Source: CAD feature listing. Evaluate the final solid. Frame: model axes, mm. A direction names the side the tool comes from. Round coordinates to 2 decimals unless told otherwise and drop trailing zeros. Order: outer loops, then holes, each group sorted by start corner. A loop starts at its lowest first (then second) coordinate and runs counter-clockwise, first axis right, second up. Notation, with made-up numbers: M -22.75,24 L 13.25,24 A22 cw 13.25,59 Z; hole C 49.5,33.5 d1. An arc over 180 degrees is marked long. Answer in a Markdown table with one row per item. Add a question column.
```python
from build123d import *

# Parameters (mm, degrees)
SKETCH1_R           = 17.5
BOSS_EXTRUDE1_DEPTH = 2
CUT_EXTRUDE2_START  = -5
CUT_EXTRUDE2_DEPTH  = 5
SKETCH4_R           = 7.5
CUT_EXTRUDE3_DEPTH  = 5
CUT_EXTRUDE5_START  = -2
CUT_EXTRUDE5_DEPTH  = 2
CIRPATTERN4_COUNT   = 9


with BuildPart() as part:
    # Sketch1 → Boss-Extrude1 (new body)
    with BuildSketch(Plane.XY):
        Circle(SKETCH1_R)
    extrude(amount=BOSS_EXTRUDE1_DEPTH)

    # Sketch3 → Cut-Extrude2 (cut)
    with BuildSketch(Plane.XY.offset(2).offset(CUT_EXTRUDE2_START)):
        with BuildLine():
            Line((12.5, -1), (17.47140521, -1))
            ThreePointArc((17.47140521, -1), (17.492849842, -0.500204374), (17.5, 0))
            ThreePointArc((17.5, 0), (17.492849842, 0.500204374), (17.47140521, 1))
            Line((17.47140521, 1), (12.5, 1))
            Line((12.5, 1), (12.5, -1))
        make_face()
    extrude(amount=CUT_EXTRUDE2_DEPTH, mode=Mode.SUBTRACT)

    # Sketch4 → Cut-Extrude3 (cut)
    with BuildSketch(Plane.XY.offset(2)):
        Circle(SKETCH4_R)
    extrude(amount=-CUT_EXTRUDE3_DEPTH, mode=Mode.SUBTRACT)

    # Sketch2 → Cut-Extrude5 (cut)
    with BuildSketch(Plane.XY.offset(2).offset(CUT_EXTRUDE5_START)):
        with BuildLine():
            Line((-17.320508076, -2.5), (-15, -2.5))
            ThreePointArc((-15, -2.5), (-13.232233047, -1.767766953), (-12.5, 0))
            ThreePointArc((-12.5, 0), (-13.232233047, 1.767766953), (-15, 2.5))
            Line((-15, 2.5), (-17.320508076, 2.5))
            ThreePointArc((-17.320508076, 2.5), (-17.5, 0), (-17.320508076, -2.5))
        make_face()
    cut_extrude5 = extrude(amount=CUT_EXTRUDE5_DEPTH, mode=Mode.SUBTRACT)

    # CirPattern4: Cut-Extrude5 ×9 about axis
    cirpattern4_axis = Axis((0, 0, 0), (0, 0, 1))
    for i in range(1, CIRPATTERN4_COUNT):
        add(cut_extrude5.rotate(cirpattern4_axis, i * 360 / CIRPATTERN4_COUNT), mode=Mode.SUBTRACT)


solid = part.part
```
(1) Line query: line 1 (Y direction, x = 6, z = 1.95); line 2 (Y direction, x = 0, z = 1.5); line 3 (Y direction, x = 1.5, z = 1.2). Output: solid intervals per line, ascending. Write a range as from..to.
(2) Cut plane A-A (y = -6.5). Return loops of the section in (x, z), and give its area (3 significant figures).
(3) Access query for faces 1 (the face through (-16, 2.5, 1)), 2 (the face through (-5.27, 15.5, 0.99)), 3 (the face through (-13.97, -8.46, 0.99)), 4 (the face through (-0.34, 16.33, 0.99)). Directions: +Z, -Z, +X, -X, +Y, -Y. A direction counts if a zero-diameter tool reaches every point of the face in a straight line with its end or side. Return the directions, or none.
(4) Cut plane B-B (x = -8). Return loops of the section in (y, z).
(5) Draft query along Y for faces 5 (the face through (-7.493, 0.33, 1.014)), 6 (the face through (-8, 0, 2)), 7 (the face through (17.35, 2.28, 0.99)). Return one class per face: +Y half, -Y half, draft (parallel to the pull), parting line (faces both ways), or undercut.
(6) Pin query (flat end, axial travel): pin 1 (1 mm diameter, centred on x = -15.5, z = 1.5, fed in from -Y); pin 2 (12 mm diameter, centred on x = 6, y = -2, fed in from -Z); pin 3 (0.6 mm diameter, centred on x = 15, z = 0.5, fed in from +Y); pin 4 (0.6 mm diameter, centred on y = 0.5, z = 1, fed in from +X). Return the tip coordinate at first contact, or that it passes through.
(7) Cut plane C-C (y = 10). Return loops of the section in (x, z), and give its area (3 significant figures).
Answer list:
| question | item | result |
|---|---|---|
| 1 | line 1 | -16.44..-15.39, -10.99..-4.5, 4.5..10.99, 15.39..16.44 |
| 1 | line 2 | -17.5..-7.5, 7.5..17.5 |
| 1 | line 3 | -17.44..-7.35, 7.35..17.44 |
| 2 | outline | M -16.25,0 L -3.74,0 L -3.74,2 L -16.25,2 Z; M 3.74,0 L 12,0 L 12,2 L 3.74,2 Z |
| 2 | area | 41.5 mm² |
| 3 | face 1 | +Z, -Z, -X |
| 3 | face 2 | +Z, -Z, +Y |
| 3 | face 3 | +Z, -Z, -Y |
| 3 | face 4 | +Z, -Z |
| 4 | outline | M -15.56,0 L 15.56,0 L 15.56,2 L -15.56,2 Z |
| 5 | face 5 | undercut |
| 5 | face 6 | draft |
| 5 | face 7 | +Y half |
| 6 | pin 1 | y = -9.01 |
| 6 | pin 2 | z = 0 |
| 6 | pin 3 | y = 9.5 |
| 6 | pin 4 | x = 12.5 |
| 7 | outline | M -9.02,0 L 14.36,0 L 14.36,2 L -9.02,2 Z |
| 7 | area | 46.8 mm² |
